```python
from build123d import *

# Parameters (mm, degrees)
BOSS_EXTRUDE1_DEPTH = 1.6
SKETCH2_R           = 3.5
BOSS_EXTRUDE2_DEPTH = 2.9
SKETCH3_R           = 2.425
CUT_EXTRUDE2_DEPTH  = 3.5
SKETCH4_R           = 1.1
CUT_EXTRUDE4_DEPTH  = 1
SKETCH5_R           = 0.5
CUT_EXTRUDE6_DEPTH  = 1.6
SKETCH6_R           = 0.5
CUT_EXTRUDE8_DEPTH  = 1.6


with BuildPart() as part:
    # Sketch1 → Boss-Extrude1 (new body)
    with BuildSketch(Plane(origin=(0, 19.3, 0), x_dir=(1, 0, 0), z_dir=(0, 1, 0))):
        with BuildLine():
            Line((5.5, -2.5), (20.5, -2.5))
            Line((20.5, -2.5), (20.5, 2.5))
            Line((20.5, 2.5), (5.5, 2.5))
            ThreePointArc((5.5, 2.5), (3, 0), (5.5, -2.5))
        make_face()
    extrude(amount=BOSS_EXTRUDE1_DEPTH)

    # Sketch2 → Boss-Extrude2 (add)
    with BuildSketch(Plane(origin=(0, 16.4, 0), x_dir=(1, 0, 0), z_dir=(0, 1, 0))):
        with Locations(Location((5.5, 0, 0), (0, 0, 45.584691403))):
            Circle(SKETCH2_R)
    extrude(amount=BOSS_EXTRUDE2_DEPTH)

    # Sketch3 → Cut-Extrude2 (cut)
    with BuildSketch(Plane(origin=(0, 16.4, 0), x_dir=(1, 0, 0), z_dir=(0, 1, 0))):
        with Locations(Location((5.5, 0, 0), (0, 0, 270))):
            Circle(SKETCH3_R)
    extrude(amount=CUT_EXTRUDE2_DEPTH, mode=Mode.SUBTRACT)

    # Sketch4 → Cut-Extrude4 (cut)
    with BuildSketch(Plane(origin=(0, 19.9, 0), x_dir=(1, 0, 0), z_dir=(0, 1, 0))):
        with Locations(Location((5.5, 0, 0), (0, 0, 270))):
            Circle(SKETCH4_R)
    extrude(amount=CUT_EXTRUDE4_DEPTH, mode=Mode.SUBTRACT)

    # Sketch5 → Cut-Extrude6 (cut)
    with BuildSketch(Plane(origin=(0, 19.3, 0), x_dir=(1, 0, 0), z_dir=(0, 1, 0))):
        with Locations(Location((15.5, 0, 0), (0, 0, 270))):
            Circle(SKETCH5_R)
    extrude(amount=CUT_EXTRUDE6_DEPTH, mode=Mode.SUBTRACT)

    # Sketch6 → Cut-Extrude8 (cut)
    with BuildSketch(Plane(origin=(0, 19.3, 0), x_dir=(1, 0, 0), z_dir=(0, 1, 0))):
        with Locations(Location((18.5, 0, 0), (0, 0, 270))):
            Circle(SKETCH6_R)
    extrude(amount=CUT_EXTRUDE8_DEPTH, mode=Mode.SUBTRACT)


solid = part.part
```
Input: part model. Units: mm. Frame: model coordinates. A direction names the side the tool comes from. Round coordinates to 2 decimals unless told otherwise and drop trailing zeros. Loops run counter-clockwise (first coordinate to the right, second up) from the corner with the lowest first, then second, coordinate; pieces in that order, holes last.
1) Set-up query: faces 5 (the flat face through (3, 19.3, 1)), 6 (the flat face through (3, 16.4, -1)), 7 (the flat face through (13, 20, 2.5)), 8 (the cylindrical face through (19, 20, 0)), 9 (the cylindrical face through (8.85, 17.83, 1.02)). Return all of +Z, -Z, +X, -X, +Y, -Y with unobstructed straight access to the full face (end or side cutting, diameter ignored); none if empty.
Ans:
face 5: -X, +Y
face 6: +Z, -Z, +X, -X, -Y
face 7: +Z, +X, -X, +Y
face 8: +Y, -Y
face 9: -Y
2) Material intervals for line 1 (X direction, y = 18.05, z = 0) (3 decimals); line 2 (Y direction, x = 12, z = -0.25); line 3 (Y direction, x = 3, z = -0.5), sorted ascending.
Ans:
line 1: x = 2 to 3.075, 7.925 to 9
line 2: y = 19.3 to 20.9
line 3: y = 16.4 to 19.3
3) Section query C-C on y = 19.65. Return the cut outline in (x, z) (3 decimals).
Ans:
outline: (5.5, -2.5) - (20.5, -2.5) - (20.5, 2.5) - (5.5, 2.5) arc R2.5 ccw to start; hole circle Ø4.85 at (5.5, 0); hole circle Ø1 at (15.5, 0); hole circle Ø1 at (18.5, 0)
4) Section query B-B on x = 4.75. Return the cut outline in (y, z), plus the area to 3 significant figures.
Ans:
outline: (16.4, -3.42) - (19.3, -3.42) - (19.3, -2.38) - (20.9, -2.38) - (20.9, -0.8) - (19.9, -0.8) - (19.9, -2.31) - (16.4, -2.31) - close; (16.4, 2.31) - (19.9, 2.31) - (19.9, 0.8) - (20.9, 0.8) - (20.9, 2.38) - (19.3, 2.38) - (19.3, 3.42) - (16.4, 3.42) - close
area: 9.71 mm2
5) Pull-direction query (X, two-part tool) for faces 1 (the cylindrical face through (3, 20.1, -0.1)), 2 (the flat face through (20.5, 20, 0)), 3 (the cylindrical face through (4.02, 18.13, -1.92)), 4 (the flat face through (12, 20.9, 0)); classes: released by +X, released by -X, zero draft, split by the parting line, or undercut.
Ans:
face 1: released by -X
face 2: released by +X
face 3: undercut
face 4: zero draft
6) Pin query (flat end, axial travel): pin 1 (1.3 mm diameter, centred on x = 9.5, y = 20.5, fed in from +Z); pin 2 (1.5 mm diameter, centred on x = 5.5, z = -0.5, fed in from -Y); pin 3 (4 mm diameter, centred on x = 12, z = 0.5, fed in from -Y). Return the tip coordinate at first contact, or that it passes through.
Ans:
pin 1: stops at z = 2.5
pin 2: stops at y = 19.9
pin 3: stops at y = 19.3
7) Section query D-D on z = -2. Return the cut outline in (x, y).
Ans:
outline: (2.63, 16.4) - (4.13, 16.4) - (4.13, 19.9) - (6.87, 19.9) - (6.87, 16.4) - (8.37, 16.4) - (8.37, 19.3) - (20.5, 19.3) - (20.5, 20.9) - (4, 20.9) - (4, 19.3) - (2.63, 19.3) - close
8) Section query A-A on z = 0. Return the cut outline in (x, y) (3 decimals), plus the area to 3 significant figures.
Ans:
outline: (2, 16.4) - (3.075, 16.4) - (3.075, 19.9) - (4.4, 19.9) - (4.4, 20.9) - (3, 20.9) - (3, 19.3) - (2, 19.3) - close; (6.6, 19.9) - (7.925, 19.9) - (7.925, 16.4) - (9, 16.4) - (9, 19.3) - (15, 19.3) - (15, 20.9) - (6.6, 20.9) - close; (16, 19.3) - (18, 19.3) - (18, 20.9) - (16, 20.9) - close; (19, 19.3) - (20.5, 19.3) - (20.5, 20.9) - (19, 20.9) - close
area: 25.9 mm2
